Check sheet for the modelled part. Datum: model origin and axes. Units: mm. A direction names the side the tool comes from. Coordinates: 2 decimals unless noted, no trailing zeros. Write each loop counter-clockwise with the first axis right and the second up, starting at its lowest first coordinate (ties: lowest second). Pieces come first, ordered by that corner, then holes. Notation, with made-up numbers: (37, 67) - (90, 67) arc R6 ccw to (90, 72) - close; hole circle Ø9 at (30.25, 24.5). An arc over 180 degrees is marked (long way). Use one line per item in the form item = value. Start each with the question number.
1. Cross-section at A-A on y = -2. Record the boundary of the cut face in (x, z), then the cut area to 3 significant figures.
2. Go/stop test with flat-tipped pins: pin 1 Ø1.6 at (y, z) = (-4, -1.5) entering from +X; pin 2 Ø2 at (x, y) = (7.5, 1.5) entering from +Z; pin 3 Ø2 at (x, z) = (2.5, -1.5) entering from -Y. Record where each tip stops, or that it passes through.
3. Draft check along Z on faces 1 (the face through (-2.822, 2.297, 12.71)), 2 (the face through (-5.985, -4.486, -0.132)), 3 (the face through (-4.4, -3.5, 0.1)), 4 (the face through (-1.365, 1.756, 6.146)). Enter one of: +Z half, -Z half, draft (parallel to the pull), parting line (faces both ways), or undercut.
4. Tool access check on faces 5 (the face through (0, -4, 0)), 6 (the face through (-2, -5.5, 0)), 7 (the face through (-3.37, 3.13, 15.18)). Record the directions out of +Z, -Z, +X, -X, +Y, -Y that give a thin tool (end or side, any length) a straight path to the whole face; none if there is none.
5. Scan lines: line 1 along X through (y, z) = (2.8, 0); line 2 along Y through (x, z) = (-15, 3). Record each from-to range of solid material in increasing order.
Autodesk Inventor part; units mm, degrees
ref_plane "YZ Plane" through (0, 0, 0) normal (1, 0, 0) x (0, 1, 0)
ref_plane "XZ Plane" through (0, 0, 0) normal (0, 1, 0) x (-1, 0, 0)
ref_plane "XY Plane" through (0, 0, 0) normal (0, 0, 1) x (1, 0, 0)
sketch "Sketch1" plane through (0, 0, 0) normal (0, 1, 0) x (-1, 0, 0)
  circle A0 centre (0, 0) radius 4
  line L0 (0, 0) -> (4, 0) construction
  line L1 (0, 0) -> (0, -4) construction
  line L2 (0, 0) -> (-4, 0) construction
  line L3 (0, 0) -> (0, 4) construction
  dimension "d0" = 8
extrude "Extrusion1" add sketch "Sketch1" against normal blind 3.5
ref_plane "Work Plane1" through (0, 0, 0) normal (0, 0, 1) x (1, 0, 0)
sketch "Sketch2" plane through (0, 0, 0) normal (0, 0, 1) x (1, 0, 0)
  line L0 (-4, 0) -> (4, 0)
  line L1 (4, 0) -> (12, 0)
  line L2 (19.05, 0.75) -> (19.05, 3)
  line L3 (17.55, 3.75) -> (15.55, 3.75)
  line L4 (0, 0) -> (0, 1.25)
  line L5 (4, 0) -> (4, 1.5959) construction
  line L6 (19.05, 0.75) -> (12, 0.75)
  line L7 (12, 0.75) -> (12, 0)
  line L8 (19.05, 3) -> (17.55, 3.75)
  line L9 (15.55, 2.5) -> (15.55, 3.75)
  line L10 (9.2263, 1.9917) -> (9.3609, 1.8771)
  line L11 (9.3609, 1.8771) -> (9.4755, 2.0117)
  line L12 (6.1006, 1.7404) -> (5.986, 1.6058)
  line L13 (5.986, 1.6058) -> (5.8514, 1.7204)
  line L14 (2.4765, 1.4491) -> (2.6111, 1.3345)
  line L15 (2.6111, 1.3345) -> (2.7257, 1.4691)
  line L16 (0, 1.25) -> (2.4765, 1.4491)
  line L17 (2.7257, 1.4691) -> (5.8514, 1.7204)
  line L18 (6.1006, 1.7404) -> (9.2263, 1.9917)
  line L19 (5.986, 1.6058) -> (5.986, 3.125) construction
  line L20 (9.3609, 1.8771) -> (9.3609, 3.125) construction
  line L21 (9.3609, 3.125) -> (5.986, 3.125) construction
  line L22 (5.986, 3.125) -> (2.6111, 3.125) construction
  line L23 (2.6111, 3.125) -> (0, 3.125) construction
  line L24 (2.4765, 1.4491) -> (2.7257, 1.4691) construction
  line L25 (5.8514, 1.7204) -> (6.1006, 1.7404) construction
  line L26 (9.2263, 1.9917) -> (9.4755, 2.0117) construction
  line L27 (2.6011, 1.4591) -> (2.6111, 1.3345) construction
  line L28 (5.986, 1.7312) -> (5.986, 1.6058) construction
  line L29 (2.6111, 1.3345) -> (2.6111, 3.125) construction
  line L30 (12.6012, 2.263) -> (12.7358, 2.1484)
  line L31 (12.7358, 2.1484) -> (12.8504, 2.283)
  line L32 (12.7358, 2.1484) -> (12.7358, 3.125) construction
  line L33 (9.4755, 2.0117) -> (12.6012, 2.263)
  line L34 (12.8504, 2.283) -> (15.55, 2.5)
  line L35 (9.3609, 3.125) -> (12.7358, 3.125) construction
  line L36 (12.7358, 3.125) -> (15.55, 3.125) construction
  point P0 (9.3609, 2.0025)
  dimension "d11" = 12
  dimension "d12" = 0.75
  dimension "d13" = 3
  dimension "d14" = 0.75
  dimension "d15" = 1.5
  dimension "d16" = 1.25
  dimension "d19" = 3.5
  dimension "d23" = 1.25
  dimension "d25" = 0.125
  dimension "d30" = 19.05
revolve "Revolution1" add sketch "Sketch2" angle 360 about axis through (0, 0, 0) along (0, 1, 0)
sketch "Sketch3" plane through (0, -3.5, 0) normal (0, -1, 0) x (1, 0, 0)
  circle A0 centre (0, 0) radius 5.986
  arc A1 (0, 5.986) -> (0, -5.986) centre (0, 0) ccw
  line L0 (0, -5.986) -> (0, 5.986)
extrude "Extrusion2" add sketch "Sketch3" along normal blind 2 contours L0 A0 picked at (-2.1196, -1.0755)
properties part number "Caps 8mm Square Rounded Caps Male"
Final values:
q1.outline = circle Ø8 at (0, 0)
q1.area = 50.3 mm²
q2.pin_1 = 3.9
q2.pin_2 = 17.91
q2.pin_3 = -3.5
q3.face_1 = undercut
q3.face_2 = parting line
q3.face_3 = draft
q3.face_4 = undercut
q4.face_5 = +Z, -Z, +X, -Y
q4.face_6 = +Z, -Z, +X, -X, -Y
q4.face_7 = +Y
q5.line_1 = -19.05 to -15.55, 15.55 to 19.05
q5.line_2 = 0.75 to 2.48
